```python
from build123d import *

# Parameters (mm, degrees)
CROQUIS1_R              = 8.25
SALIENTE_EXTRUIR1_DEPTH = 3


with BuildPart() as part:
    # Croquis1 → Saliente-Extruir1 (new body)
    with BuildSketch(Plane.XY):
        Polygon((-175, -97), (-165, -97), (-165, -100), (-155, -100), (-155, -97), (-145, -97), (-145, -100), (-135, -100), (-135, -97), (-125, -97), (-125, -100), (-115, -100), (-115, -97), (-105, -97), (-105, -100), (-95, -100), (-95, -97), (-85, -97), (-85, -100), (-75, -100), (-75, -97), (-65, -97), (-65, -100), (-55, -100), (-55, -97), (-45, -97), (-45, -100), (-35, -100), (-35, -97), (-25, -97), (-25, -100), (-15, -100), (-15, -97), (-5, -97), (-5, -100), (5, -100), (5, -97), (15, -97), (15, -100), (25, -100), (25, -97), (35, -97), (35, -100), (45, -100), (45, -97), (55, -97), (55, -100), (65, -100), (65, -97), (75, -97), (75, -100), (85, -100), (85, -97), (95, -97), (95, -100), (105, -100), (105, -97), (115, -97), (115, -100), (125, -100), (125, -97), (135, -97), (135, -100), (145, -100), (145, -97), (155, -97), (155, -100), (165, -100), (165, -97), (175, -97), (175, -90), (172, -90), (172, -80), (175, -80), (175, -70), (172, -70), (172, -60), (175, -60), (175, -50), (172, -50), (172, -40), (175, -40), (175, -30), (172, -30), (172, -20), (175, -20), (175, -10), (172, -10), (172, 0), (175, 0), (175, 10), (172, 10), (172, 20), (175, 20), (175, 30), (172, 30), (172, 40), (175, 40), (175, 50), (172, 50), (172, 60), (175, 60), (175, 70), (172, 70), (172, 80), (175, 80), (175, 90), (172, 90), (172, 97), (165, 97), (165, 100), (155, 100), (155, 97), (145, 97), (145, 100), (135, 100), (135, 97), (125, 97), (125, 100), (115, 100), (115, 97), (105, 97), (105, 100), (95, 100), (95, 97), (85, 97), (85, 100), (75, 100), (75, 97), (65, 97), (65, 100), (55, 100), (55, 97), (45, 97), (45, 100), (35, 100), (35, 97), (25, 97), (25, 100), (15, 100), (15, 97), (5, 97), (5, 100), (-5, 100), (-5, 97), (-15, 97), (-15, 100), (-25, 100), (-25, 97), (-35, 97), (-35, 100), (-45, 100), (-45, 97), (-55, 97), (-55, 100), (-65, 100), (-65, 97), (-75, 97), (-75, 100), (-85, 100), (-85, 97), (-95, 97), (-95, 100), (-105, 100), (-105, 97), (-115, 97), (-115, 100), (-125, 100), (-125, 97), (-135, 97), (-135, 100), (-145, 100), (-145, 97), (-155, 97), (-155, 100), (-165, 100), (-165, 97), (-172, 97), (-172, 90), (-175, 90), (-175, 80), (-172, 80), (-172, 70), (-175, 70), (-175, 60), (-172, 60), (-172, 50), (-175, 50), (-175, 40), (-172, 40), (-172, 30), (-175, 30), (-175, 20), (-172, 20), (-172, 10), (-175, 10), (-175, 0), (-172, 0), (-172, -10), (-175, -10), (-175, -20), (-172, -20), (-172, -30), (-175, -30), (-175, -40), (-172, -40), (-172, -50), (-175, -50), (-175, -60), (-172, -60), (-172, -70), (-175, -70), (-175, -80), (-172, -80), (-172, -90), (-175, -90), align=None)
        with Locations((-13, 0)):
            Circle(CROQUIS1_R, mode=Mode.SUBTRACT)
        with Locations((13, 0)):
            Circle(CROQUIS1_R, mode=Mode.SUBTRACT)
    extrude(amount=SALIENTE_EXTRUIR1_DEPTH)


solid = part.part
```
Check sheet for the modelled part. Datum: model origin and axes. Units: mm. Round coordinates to 2 decimals unless told otherwise and drop trailing zeros. Loops run counter-clockwise (first coordinate to the right, second up) from the corner with the lowest first, then second, coordinate; pieces in that order, holes last. Notation, with made-up numbers: (36, 56) -> (45, 56) arc R12 cw to (45, 61) -> close; hole circle Ø3 at (-3, -37.75). An arc over 180 degrees is marked (long way). Write item = value, one per line. Start each with the question number.
1) Sectioned sample at C-C, the plane y = 35. Record the cut outline in (x, z), plus the area to 3 significant figures.
2) Thickness scan on probe 1 along Y at (x, z) = (13, 1.3); probe 2 along X at (y, z) = (-88, 0.4); probe 3 along Y at (x, z) = (-67.5, 2.65). Record the ranges inside material, lowest first.
3) Sectioned sample at B-B, the plane z = 2.05. State how many separate pieces and enclosed holes the cut face has, plus the area to 3 significant figures.
4) Sectioned sample at A-A, the plane x = 70. Record the cut outline in (y, z), plus the area to 3 significant figures.
5) Release check for a two-part mould opening along Y. For faces 1 (the flat face through (-2, 1, 3)), 2 (the cylindrical face through (20.87, 2.48, 1.48)) record: released by +Y, released by -Y, zero draft, split by the parting line, or undercut.
6) Gauge pin test, flat ends, axial feed: pin 1 Ø1.5 at (x, z) = (173.5, 1) entering from -Y; pin 2 Ø1.5 at (y, z) = (98, 1.5) entering from -X; pin 3 Ø1.5 at (x, z) = (-174, 1.5) entering from +Y. Record the tip position at first contact, or that the pin passes through.
Results are:
q1.outline = (-172, 0) -> (172, 0) -> (172, 3) -> (-172, 3) -> close
q1.area = 1,030 mm^2
q2.probe_1 = -97 to -8.25, 8.25 to 97
q2.probe_2 = -172 to 172
q2.probe_3 = -97 to 97
q3.separate_pieces = 1
q3.enclosed_holes = 2
q3.area = 67,900 mm^2
q4.outline = (-97, 0) -> (97, 0) -> (97, 3) -> (-97, 3) -> close
q4.area = 582 mm^2
q5.face_1 = zero draft
q5.face_2 = undercut
q6.pin_1 = -97
q6.pin_2 = -165
q6.pin_3 = 90
